Input: part model. Units: mm. Frame: model coordinates. A direction names the side the tool comes from. Round coordinates to 2 decimals unless told otherwise and drop trailing zeros. Order: outer loops, then holes, each group sorted by start corner. A loop starts at its lowest first (then second) coordinate and runs counter-clockwise, first axis right, second up. Notation, with made-up numbers: (13, 31.25) -> (57, 31.25) arc R11 cw to (57, 50.25) -> close; hole circle Ø3 at (54, 4). An arc over 180 degrees is marked (long way). Use a Markdown table: item, result.
from build123d import *

# Parameters (mm, degrees)
SKETCH_R        = 15
PAD_DEPTH       = 20
SKETCH003_W     = 20
SKETCH003_H     = 40
PAD002_DEPTH    = 20
SKETCH002_R     = 3
POCKET_DEPTH    = 20.001
POCKET001_DEPTH = 20.001
SKETCH005_R     = 5.1
POCKET002_DEPTH = 20.001


with BuildPart() as part:
    # Sketch → Pad (new body, symmetric)
    with BuildSketch(Plane.XY):
        Circle(SKETCH_R)
    extrude(amount=PAD_DEPTH, both=True)

    # Sketch003 → Pad002 (join)
    with BuildSketch(Plane.XZ):
        Rectangle(SKETCH003_W, SKETCH003_H)
    extrude(amount=-PAD002_DEPTH)

    # Sketch002 → Pocket (cut, through all)
    with BuildSketch(Plane.XZ):
        with Locations((0, 10)):
            Circle(SKETCH002_R)
        with Locations((0, -10)):
            Circle(SKETCH002_R)
    extrude(amount=-POCKET_DEPTH, mode=Mode.SUBTRACT)

    # Sketch004 → Pocket001 (cut, through all)
    with BuildSketch(Plane.XY):
        with BuildLine():
            ThreePointArc((-4.781213, 5.45), (0, -7.25), (4.781213, 5.45))
            Line((-4.781213, 5.45), (4.781213, 5.45))
        make_face()
    extrude(amount=-POCKET001_DEPTH, mode=Mode.SUBTRACT)

    # Sketch005 → Pocket002 (cut, through all)
    with BuildSketch(Plane.XY):
        Circle(SKETCH005_R)
    extrude(amount=POCKET002_DEPTH, mode=Mode.SUBTRACT)


solid = part.part
1) Cut plane A-A on x = 0. Return loops of the section in (y, z), and give its area (3 significant figures).
Results found:
| item | result |
|---|---|
| outline | (-15, -20) -> (-7.25, -20) -> (-7.25, 0) -> (-5.1, 0) -> (-5.1, 20) -> (-15, 20) -> close; (5.1, 0) -> (5.45, 0) -> (5.45, -7) -> (20, -7) -> (20, 7) -> (5.1, 7) -> close; (5.1, 13) -> (20, 13) -> (20, 20) -> (5.1, 20) -> close; (5.45, -20) -> (20, -20) -> (20, -13) -> (5.45, -13) -> close |
| area | 765 mm² |
2) Pin query (flat end, axial travel): pin 1 Ø1 at (y, z) = (-9.5, -6) entering from -X; pin 2 Ø7 at (y, z) = (16.5, 8.5) entering from +X; pin 3 Ø6 at (y, z) = (7, 12.5) entering from +X; pin 4 Ø8 at (x, y) = (0, 0) entering from -Z. Return the tip coordinate at first contact, or that it passes through.
Results found:
| item | result |
|---|---|
| pin 1 | stops at x = -12 |
| pin 2 | stops at x = 10 |
| pin 3 | stops at x = 14.46 |
| pin 4 | passes through |
3) Cut plane D-D on x = -3.75. Return loops of the section in (y, z).
Results found:
| item | result |
|---|---|
| outline | (-14.52, -20) -> (-6.2, -20) -> (-6.2, 0) -> (-3.46, 0) -> (-3.46, 20) -> (-14.52, 20) -> close; (3.46, 0) -> (5.45, 0) -> (5.45, -20) -> (20, -20) -> (20, 20) -> (3.46, 20) -> close |
4) Cut plane C-C on z = 10. Return loops of the section in (x, y), and give its area (3 significant figures).
Results found:
| item | result |
|---|---|
| outline | (-10, 11.18) arc R15 ccw (long way) to (10, 11.18) -> (10, 20) -> (3, 20) -> (3, 4.12) arc R5.1 cw (long way) to (-3, 4.12) -> (-3, 20) -> (-10, 20) -> close |
| area | 658 mm² |
5) Line query: L1, parallel to Z at x = 0, y = 9.25; L2, parallel to Y at x = 0, z = 15.25; L3, parallel to X at y = 13, z = 10. Output: solid intervals per line, ascending. Write a range as [from, to].
Results found:
| item | result |
|---|---|
| L1 | z = [-20, -13], [-7, 7], [13, 20] |
| L2 | y = [-15, -5.1], [5.1, 20] |
| L3 | x = [-10, -3], [3, 10] |
6) Cut plane B-B on z = -16.5. Return loops of the section in (x, y), and give its area (3 significant figures).
Results found:
| item | result |
|---|---|
| outline | (-10, 11.18) arc R15 ccw (long way) to (10, 11.18) -> (10, 20) -> (-10, 20) -> close; hole (-4.78, 5.45) arc R7.25 ccw (long way) to (4.78, 5.45) -> close |
| area | 678 mm² |
7) Pull-direction query (Y, two-part tool) for faces 1 (the flat face through (2, -5, 0)), 2 (the flat face through (0, 20, 0)), 3 (the cylindrical face through (0, 13, -7)), 4 (the cylindrical face through (-0.246, -7.246, -9.86)); classes: +Y half, -Y half, draft (parallel to the pull), parting line (faces both ways), or undercut.
Results found:
| item | result |
|---|---|
| face 1 | undercut |
| face 2 | +Y half |
| face 3 | draft |
| face 4 | undercut |
8) Set-up query: faces 5 (the cylindrical face through (0, 12, 13)), 6 (the flat face through (10, 16, 0)), 7 (the flat face through (-10, 16, 0)), 8 (the flat face through (-2.2, 5.45, -7.6)). Return all of +Z, -Z, +X, -X, +Y, -Y with unobstructed straight access to the full face (end or side cutting, diameter ignored); none if empty.
Results found:
| item | result |
|---|---|
| face 5 | +Y |
| face 6 | +Z, -Z, +X, +Y |
| face 7 | +Z, -Z, -X, +Y |
| face 8 | -Z |
